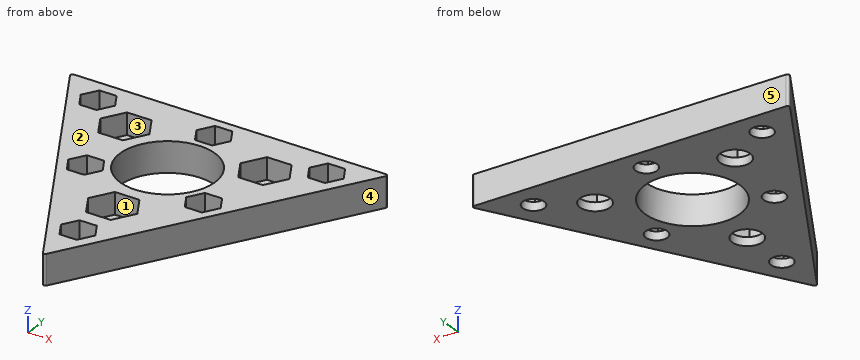
from build123d import *

# Parameters (mm, degrees)
F0_R     = 11
F1_DEPTH = 7
F2_R     = 0.5
F0_R_2   = 2.5
F0_R_3   = 3.5
F3_DEPTH = 2


with BuildPart() as f1:
    # F0 (on Top) → F1 (new body)
    with BuildSketch(Plane.XY):
        Polygon((0, -43.30127), (37.5, 21.650635), (-37.5, 21.650635), align=None)
        Polygon((4.041452, -31), (2.020726, -34.5), (-2.020726, -34.5), (-4.041452, -31), (-2.020726, -27.5), (2.020726, -27.5), align=None, mode=Mode.SUBTRACT)
        Polygon((2.886751, -14), (5.773503, -19), (2.886751, -24), (-2.886751, -24), (-5.773503, -19), (-2.886751, -14), align=None, mode=Mode.SUBTRACT)
        Polygon((-9.814955, -8), (-11.835681, -11.5), (-15.877132, -11.5), (-17.897858, -8), (-15.877132, -4.5), (-11.835681, -4.5), align=None, mode=Mode.SUBTRACT)
        Polygon((-22.805336, 15.5), (-24.826062, 12), (-28.867513, 12), (-30.888239, 15.5), (-28.867513, 19), (-24.826062, 19), align=None, mode=Mode.SUBTRACT)
        Polygon((-13.567731, 4.5), (-19.341234, 4.5), (-22.227985, 9.5), (-19.341234, 14.5), (-13.567731, 14.5), (-10.68098, 9.5), align=None, mode=Mode.SUBTRACT)
        Polygon((9.814955, -8), (11.835681, -4.5), (15.877132, -4.5), (17.897858, -8), (15.877132, -11.5), (11.835681, -11.5), align=None, mode=Mode.SUBTRACT)
        Circle(F0_R, mode=Mode.SUBTRACT)
        Polygon((22.227985, 9.5), (19.341234, 4.5), (13.567731, 4.5), (10.68098, 9.5), (13.567731, 14.5), (19.341234, 14.5), align=None, mode=Mode.SUBTRACT)
        Polygon((-2.020726, 19.5), (2.020726, 19.5), (4.041452, 16), (2.020726, 12.5), (-2.020726, 12.5), (-4.041452, 16), align=None, mode=Mode.SUBTRACT)
        Polygon((30.888239, 15.5), (28.867513, 12), (24.826062, 12), (22.805336, 15.5), (24.826062, 19), (28.867513, 19), align=None, mode=Mode.SUBTRACT)
    extrude(amount=F1_DEPTH)

    # F2
    f2_edges = [f1.edges().sort_by_distance(p)[0] for p in [
        (0, -43.30127, 3.5),
        (-37.5, 21.650635, 3.5),
        (37.5, 21.650635, 3.5),
    ]]
    fillet(f2_edges, radius=F2_R)

    # F0 (on Top) → F3 (join)
    with BuildSketch(Plane.XY):
        Polygon((4.041452, 16), (2.020726, 19.5), (-2.020726, 19.5), (-4.041452, 16), (-2.020726, 12.5), (2.020726, 12.5), align=None)
        with Locations((0, 16)):
            Circle(F0_R_2, mode=Mode.SUBTRACT)
        Polygon((-22.227985, 9.5), (-19.341234, 4.5), (-13.567731, 4.5), (-10.68098, 9.5), (-13.567731, 14.5), (-19.341234, 14.5), align=None)
        with Locations((-16.454483, 9.5)):
            Circle(F0_R_3, mode=Mode.SUBTRACT)
        Polygon((-15.877132, -11.5), (-11.835681, -11.5), (-9.814955, -8), (-11.835681, -4.5), (-15.877132, -4.5), (-17.897858, -8), align=None)
        with Locations((-13.856406, -8)):
            Circle(F0_R_2, mode=Mode.SUBTRACT)
        Polygon((-28.867513, 12), (-24.826062, 12), (-22.805336, 15.5), (-24.826062, 19), (-28.867513, 19), (-30.888239, 15.5), align=None)
        with Locations((-26.846788, 15.5)):
            Circle(F0_R_2, mode=Mode.SUBTRACT)
        Polygon((2.886751, -24), (5.773503, -19), (2.886751, -14), (-2.886751, -14), (-5.773503, -19), (-2.886751, -24), align=None)
        with Locations((0, -19)):
            Circle(F0_R_3, mode=Mode.SUBTRACT)
        Polygon((-2.020726, -34.5), (2.020726, -34.5), (4.041452, -31), (2.020726, -27.5), (-2.020726, -27.5), (-4.041452, -31), align=None)
        with Locations((0, -31)):
            Circle(F0_R_2, mode=Mode.SUBTRACT)
        Polygon((15.877132, -4.5), (11.835681, -4.5), (9.814955, -8), (11.835681, -11.5), (15.877132, -11.5), (17.897858, -8), align=None)
        with Locations((13.856406, -8)):
            Circle(F0_R_2, mode=Mode.SUBTRACT)
        Polygon((13.567731, 4.5), (19.341234, 4.5), (22.227985, 9.5), (19.341234, 14.5), (13.567731, 14.5), (10.68098, 9.5), align=None)
        with Locations((16.454483, 9.5)):
            Circle(F0_R_3, mode=Mode.SUBTRACT)
        Polygon((24.826062, 12), (28.867513, 12), (30.888239, 15.5), (28.867513, 19), (24.826062, 19), (22.805336, 15.5), align=None)
        with Locations((26.846788, 15.5)):
            Circle(F0_R_2, mode=Mode.SUBTRACT)
    extrude(amount=F3_DEPTH)


solid = f1.part
Work out the finished part from the listing and answer in its coordinate system (mm). Face numbers are marked on the shaded views. A direction names the side the tool comes from. Coordinates: 2 decimals unless noted, no trailing zeros. Order: outer loops, then holes, each group sorted by start corner. A loop starts at its lowest first (then second) coordinate and runs counter-clockwise, first axis right, second up. Notation, with made-up numbers: (-0.75, 62) - (46.25, 62) arc R17 cw to (46.25, 67) - close; hole circle Ø2 at (62.5, -11). An arc over 180 degrees is marked (long way). Put each result on its own line as item: value. Start each with the question number.
1) Find the intervals of material crossed by line 1 (X direction, y = 16, z = 4.25); line 2 (Y direction, x = -12.5, z = 3); line 3 (X direction, y = -9, z = 0.5), in increasing order. Write a range as from..to.
2) Find section B-B (x = -33). Give the vertices of the cut face in (y, z), plus the area to 3 significant figures.
3) Find section A-A (y = 0). Give the vertices of the cut face in (x, z), plus the area to 3 significant figures.
4) For the marked faces 1 and 2, determine the directions among +Z, -Z, +X, -X, +Y, -Y from which every point of the face is accessible in a straight line to the end or side of a thin tool.
5) For a pull along X with two mould halves and no side action, classify the marked faces 3, 4 and 5 as released by +X, released by -X, zero draft, split by the parting line, or undercut.
6) Flat-ended cylindrical pins translate along their axes: pin 1 (3 mm diameter, centred on x = 14.5, y = 7, fed in from +Z); pin 2 (4.5 mm diameter, centred on x = 0, y = -31, fed in from -Z); pin 3 (1.5 mm diameter, centred on x = 28, z = 5, fed in from -Y); pin 4 (1.2 mm diameter, centred on x = 13, z = 5.5, fed in from -Y). Find the tip coordinate at first contact, or state that the pin passes through.
Results list:
1. line 1: x = -34.24..-30.6, -23.09..-4.04, 4.04..23.09, 30.6..34.24
1. line 2: y = -21.65..-11.5, -4.5..6.35, 12.65..21.65
1. line 3: x = -19.8..-16.15, -11.57..-6.32, 6.32..11.57, 16.15..19.8
2. outline: (13.86, 0) - (21.65, 0) - (21.65, 7) - (13.86, 7) - close
2. area: 54.6 mm^2
3. outline: (-25, 0) - (-11, 0) - (-11, 7) - (-25, 7) - close; (11, 0) - (25, 0) - (25, 7) - (11, 7) - close
3. area: 196 mm^2
4. face 1: +Z
4. face 2: +Z, +X, -X, +Y, -Y
5. face 3: undercut
5. face 4: released by +X
5. face 5: zero draft
6. pin 1: stops at z = 2
6. pin 2: passes through
6. pin 3: stops at y = 3.9
6. pin 4: stops at y = -21.82
